The listing builds one solid part. Answer for the finished solid, in the listing's coordinates (mm). Face numbers are marked on the shaded views. A direction names the side the tool comes from. Round coordinates to 2 decimals unless told otherwise and drop trailing zeros. Write each loop counter-clockwise with the first axis right and the second up, starting at its lowest first coordinate (ties: lowest second). Pieces come first, ordered by that corner, then holes. Notation, with made-up numbers: (34.5, 49) - (63.5, 49) arc R19 ccw to (63.5, 77) - close; hole circle Ø6 at (61.5, 79). An arc over 180 degrees is marked (long way). Answer in a Markdown table with one row per item.
Autodesk Inventor part; units mm, degrees
ref_plane "YZ Plane" through (0, 0, 0) normal (1, 0, 0) x (0, 1, 0)
ref_plane "XZ Plane" through (0, 0, 0) normal (0, 1, 0) x (-1, 0, 0)
ref_plane "XY Plane" through (0, 0, 0) normal (0, 0, 1) x (1, 0, 0)
sketch "Sketch1" plane through (0, 0, 0) normal (0, 0, 1) x (1, 0, 0)
  line L0 (-8.995, 0) -> (8.995, 0)
  arc A0 (8.995, 0) -> (8.995, 5) centre (8.995, 2.5) ccw
  arc A1 (-8.995, 5) -> (-8.995, 0) centre (-8.995, 2.5) ccw
  line L1 (-8.995, 0) -> (-8.995, 5) construction
  line L2 (8.995, 0) -> (8.995, 5) construction
  arc A2 (8.995, 30) -> (8.6755, 34.9795) centre (8.995, 32.5) ccw
  arc A3 (-8.6755, 34.9795) -> (-8.995, 30) centre (-8.995, 32.5) ccw
  line L3 (-1.5, 19) -> (1.5, 19)
  line L4 (1.5, 19) -> (1.5, 16)
  line L5 (1.5, 16) -> (-1.5, 16)
  line L6 (-1.5, 16) -> (-1.5, 19)
  line L7 (-1.5, 19) -> (1.5, 16) construction
  line L8 (1.5, 19) -> (-1.5, 16) construction
  line L9 (-8.995, 35.0339) -> (-8.995, 30) construction
  line L10 (8.995, 35.0339) -> (8.995, 30) construction
  line L11 (-5.0276, 26.51) -> (5.0276, 26.51) construction
  line L12 (5.0276, 26.51) -> (5.0276, 8.49)
  line L13 (5.0276, 8.49) -> (-5.0276, 8.49) construction
  line L14 (-5.0276, 8.49) -> (-5.0276, 26.51)
  line L15 (-5.0276, 26.51) -> (5.0276, 8.49) construction
  line L16 (5.0276, 26.51) -> (-5.0276, 8.49) construction
  arc A4 (8.995, 30) -> (5.0276, 26.51) centre (8.995, 26) ccw
  arc A5 (-5.0276, 26.51) -> (-8.995, 30) centre (-8.995, 26) ccw
  arc A6 (-8.995, 5) -> (-5.0276, 9.51) centre (-8.995, 9) ccw
  arc A7 (5.0276, 8.49) -> (8.995, 5) centre (8.995, 9) ccw
  arc A8 (5, 36.5) -> (-5, 36.5) centre (0, 36.5) ccw
  line L17 (-5, 36.5) -> (5, 36.5) construction
  arc A9 (-8.995, 35.0339) -> (-5, 36.5) centre (-8.1644, 38.9467) ccw
  arc A10 (5, 36.5) -> (8.995, 35.0339) centre (8.1644, 38.9467) ccw
  circle A11 centre (0, 36.5) radius 1.5
  point P0 (0, 0)
  point P1 (-8.995, 2.5)
  point P2 (8.995, 2.5)
  point P3 (0, 17.5)
  point P4 (-11.495, 32.5)
  point P5 (-11.495, 2.5)
  point P6 (0, 41.5)
  point P7 (11.495, 32.5)
  point P8 (11.495, 2.5)
  point P9 (-8.995, 32.5169)
  dimension "d1" = 2.5
  dimension "d2" = 2.5
  dimension "d3" = 2.5
  dimension "d4" = 32.5
  dimension "d6" = 3
  dimension "d7" = 3
  dimension "d8" = 16
  dimension "d12" = 18.02
  dimension "d13" = 4
  dimension "d14" = 4
  dimension "d16" = 5
  dimension "d17" = 4
  dimension "d22" = 41.5
  dimension "d25" = 22.99
  dimension "d29" = 3
  dimension "d30" = 36.5
  dimension "d33" = 8.995
extrude "Extrusion1" add sketch "Sketch1" along normal blind 3 contours A1 A6 L14 A5 A3 A9 A8 A10 A2 A4 L12 A7 A0 L0
sketch "Sketch2" plane through (0, 0, 3) normal (0, 0, 1) x (1, 0, 0)
  arc A0 (8.995, 30) -> (8.6755, 34.9795) centre (8.995, 32.5) ccw
  arc A1 (-8.6755, 34.9795) -> (-8.995, 30) centre (-8.995, 32.5) ccw
  arc A2 (-8.995, 5) -> (-8.995, 0) centre (-8.995, 2.5) ccw
  arc A3 (8.995, 0) -> (8.995, 5) centre (8.995, 2.5) ccw
  point P0 (0, 0)
hole "Hole1" at (-8.995, 32.5, 3) at (8.995, 32.5, 3) at (8.995, 2.5, 3) at (-8.995, 2.5, 3) direction (0, 0, -1) diameter 1.567 end through all
properties part number "23 - Valve Disc" material "Steel AISI 1020 107 HR"
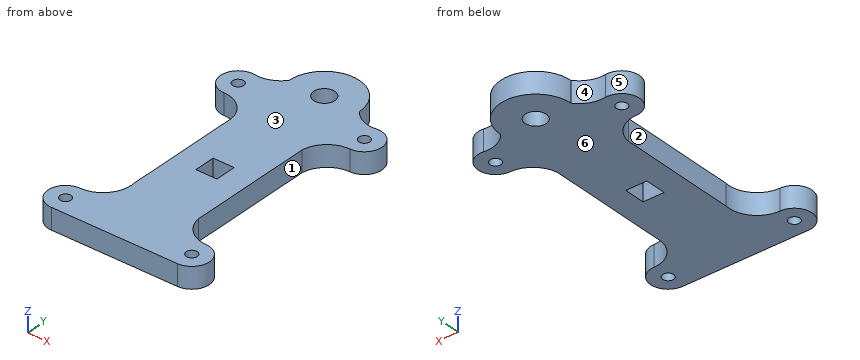
(1) For the marked faces 1, 2 and 3, determine the directions among +Z, -Z, +X, -X, +Y, -Y from which every point of the face is accessible in a straight line to the end or side of a thin tool.
Checked values:
| item | result |
|---|---|
| face 1 | +Z, -Z, +X |
| face 2 | +Z, -Z, -X |
| face 3 | +Z, +X, -X, +Y, -Y |
(2) For a pull along Y with two mould halves and no side action, classify the marked faces 4, 5 and 6 as pulls with the +Y half, pulls with the -Y half, needs draft (parallel to the pull), parting line crosses it, or undercut.
Checked values:
| item | result |
|---|---|
| face 4 | pulls with the +Y half |
| face 5 | undercut |
| face 6 | needs draft |
(3) Section B-B (x = -7.5) is taken. Give the vertices of the cut face in (y, z).
Checked values:
| item | result |
|---|---|
| outline | (0, 0) - (5.29, 0) - (5.29, 3) - (0, 3) - close; (29.71, 0) - (35, 0) - (35, 3) - (29.71, 3) - close |
(4) Section A-A (y = 32.5) is taken. Give the vertices of the cut face in (x, z) (1 decimal), and give its area (3 significant figures).
Checked values:
| item | result |
|---|---|
| outline | (-11.5, 0) - (-9.8, 0) - (-9.8, 3) - (-11.5, 3) - close; (-8.2, 0) - (8.2, 0) - (8.2, 3) - (-8.2, 3) - close; (9.8, 0) - (11.5, 0) - (11.5, 3) - (9.8, 3) - close |
| area | 59.6 mm2 |
(5) Section D-D (y = 11.5) is taken. Give the vertices of the cut face in (x, z), and give its area (3 significant figures).
Checked values:
| item | result |
|---|---|
| outline | (-5.03, 0) - (5.03, 0) - (5.03, 3) - (-5.03, 3) - close |
| area | 30.2 mm2 |
(6) Section C-C (z = 1.85) is taken. Give the vertices of the cut face in (x, y) (1 decimal), and give its area (3 significant figures).
Checked values:
| item | result |
|---|---|
| outline | (-9, 0) - (9, 0) arc R2.5 ccw to (9, 5) arc R4 cw to (5, 8.5) - (5, 26.5) arc R4 cw to (9, 30) arc R2.5 ccw (long way) to (8.7, 35) arc R4 cw to (5, 36.5) arc R5 ccw to (-5, 36.5) arc R4 cw to (-8.7, 35) arc R2.5 ccw (long way) to (-9, 30) arc R4 cw to (-5, 26.5) - (-5, 9.5) arc R4 cw to (-9, 5) arc R2.5 ccw to start; hole circle Ø1.6 at (-9, 2.5); hole circle Ø1.6 at (-9, 32.5); hole (-1.5, 16) - (1.5, 16) - (1.5, 19) - (-1.5, 19) - close; hole circle Ø3 at (0, 36.5); hole circle Ø1.6 at (9, 2.5); hole circle Ø1.6 at (9, 32.5) |
| area | 517 mm2 |
(7) Find the intervals of material crossed by line 1 (Y direction, x = 0, z = 1.25); line 2 (X direction, y = 2.5, z = 0.8) (1 decimal); line 3 (X direction, y = 13, z = 0.1), in increasing order.
Checked values:
| item | result |
|---|---|
| line 1 | y = 0 to 16, 19 to 35, 38 to 41.5 |
| line 2 | x = -11.5 to -9.8, -8.2 to 8.2, 9.8 to 11.5 |
| line 3 | x = -5.03 to 5.03 |
(8) Flat-ended cylindrical pins translate along their axes: pin 1 (1.3 mm diameter, centred on x = 8.995, y = 2.5, fed in from +Z); pin 2 (1 mm diameter, centred on x = 3, z = 1, fed in from +Y); pin 3 (1.5 mm diameter, centred on y = 18, z = 2, fed in from +X). Find the tip coordinate at first contact, or state that the pin passes through.
Checked values:
| item | result |
|---|---|
| pin 1 | passes through |
| pin 2 | stops at y = 40.83 |
| pin 3 | stops at x = 5.03 |
